The model under review builds one solid part; all positions refer to its coordinate system, in mm. Coordinates: 2 decimals unless noted, no trailing zeros. Write each loop counter-clockwise with the first axis right and the second up, starting at its lowest first coordinate (ties: lowest second). Pieces come first, ordered by that corner, then holes. Notation, with made-up numbers: (36.5, 86) -> (55.5, 86) arc R12 ccw to (55.5, 95) -> close; hole circle Ø9 at (89.5, 86). An arc over 180 degrees is marked (long way). Write each question's results on one line, items separated by ' | '.
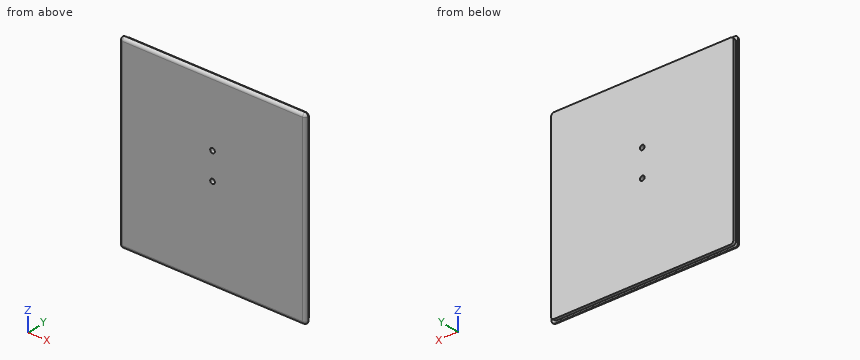
```python
from build123d import *

# Parameters (mm, degrees)
SKETCH1_W           = 120
SKETCH1_H           = 120
BOSS_EXTRUDE1_DEPTH = 2
SKETCH2_W           = 117.5
SKETCH2_H           = 117.5
BOSS_EXTRUDE2_DEPTH = 2
FILLET1_R           = 2
SKETCH4_R           = 1.5
CUT_EXTRUDE1_DEPTH  = 85.947042326


with BuildPart() as part:
    # Sketch1 → Boss-Extrude1 (new body)
    with BuildSketch(Plane(origin=(0, 0, 0), x_dir=(1, 0, 0), z_dir=(0, 1, 0))):
        Rectangle(SKETCH1_W, SKETCH1_H)
    extrude(amount=BOSS_EXTRUDE1_DEPTH)

    # Sketch2 → Boss-Extrude2 (add)
    with BuildSketch(Plane(origin=(0, 2, 0), x_dir=(1, 0, 0), z_dir=(0, 1, 0))):
        Rectangle(SKETCH2_W, SKETCH2_H)
    extrude(amount=BOSS_EXTRUDE2_DEPTH)

    # Fillet1
    fillet1_edges = [part.edges().sort_by_distance(p)[0] for p in [
        (58.75, 3, 58.75),
        (58.75, 3, -58.75),
        (-58.75, 3, -58.75),
        (-58.75, 3, 58.75),
        (0, 0, 60),
        (-60, 0, 0),
        (0, 0, -60),
        (60, 0, 0),
        (60, 1, 60),
        (-60, 1, 60),
        (-60, 1, -60),
        (60, 1, -60),
    ]]
    fillet(fillet1_edges, radius=FILLET1_R - 0.0001)  # a hair under: the kernel refuses the full size

    # Sketch4 → Cut-Extrude1 (cut, through all)
    with BuildSketch(Plane.XZ):
        with Locations(Location((0, 0, 0), (0, 0, 270))):
            Circle(SKETCH4_R)
        with Locations(Location((0, 17.5, 0), (0, 0, 270))):
            Circle(SKETCH4_R)
    extrude(amount=-CUT_EXTRUDE1_DEPTH, mode=Mode.SUBTRACT)


solid = part.part
```
Q1. Add section B-B (x = 0). Count the separate pieces of the cut face and the enclosed holes in it, plus the area to 3 significant figures.
Solution:
separate pieces: 3 | enclosed holes: 0 | area: 449 mm²
Q2. Clearance check with flat-ended pins moving along their axes: P1, Ø1.6, axis at y = 3, z = -1, coming from the -X side; P2, Ø2.5, axis at x = 0, z = 17.5, coming from the -Y side; P3, Ø1.6, axis at x = 5, y = 3, coming from the +Z side; P4, Ø1.5, axis at x = 16.5, y = 1, coming from the +Z side. State where each tip first meets the part, or that it passes through.
Solution:
P1: x = -58.75 | P2: through | P3: z = 58.75 | P4: z = 59.98
Q3. For line 1 (X direction, y = 3.2, z = 17.5); line 2 (X direction, y = 1.75, z = 17.5); line 3 (X direction, y = 2.1, z = 49.5), list the stretches that pass through material, from the lowest coordinate up. Write a range as from..to.
Solution:
line 1: -58.75..-1.5, 1.5..58.75 | line 2: -59.98..-1.5, 1.5..59.98 | line 3: -58.75..58.75
Q4. Add section C-C (y = 0.6). Write out the cut boundary in (x, z), plus the area to 3 significant figures.
Solution:
outline: (-59.43, -58) arc R1.43 ccw to (-58, -59.43) -> (58, -59.43) arc R1.43 ccw to (59.43, -58) -> (59.43, 58) arc R1.43 ccw to (58, 59.43) -> (-58, 59.43) arc R1.43 ccw to (-59.43, 58) -> close; hole circle Ø3 at (0, 0); hole circle Ø3 at (0, 17.5) | area: 14,100 mm²
